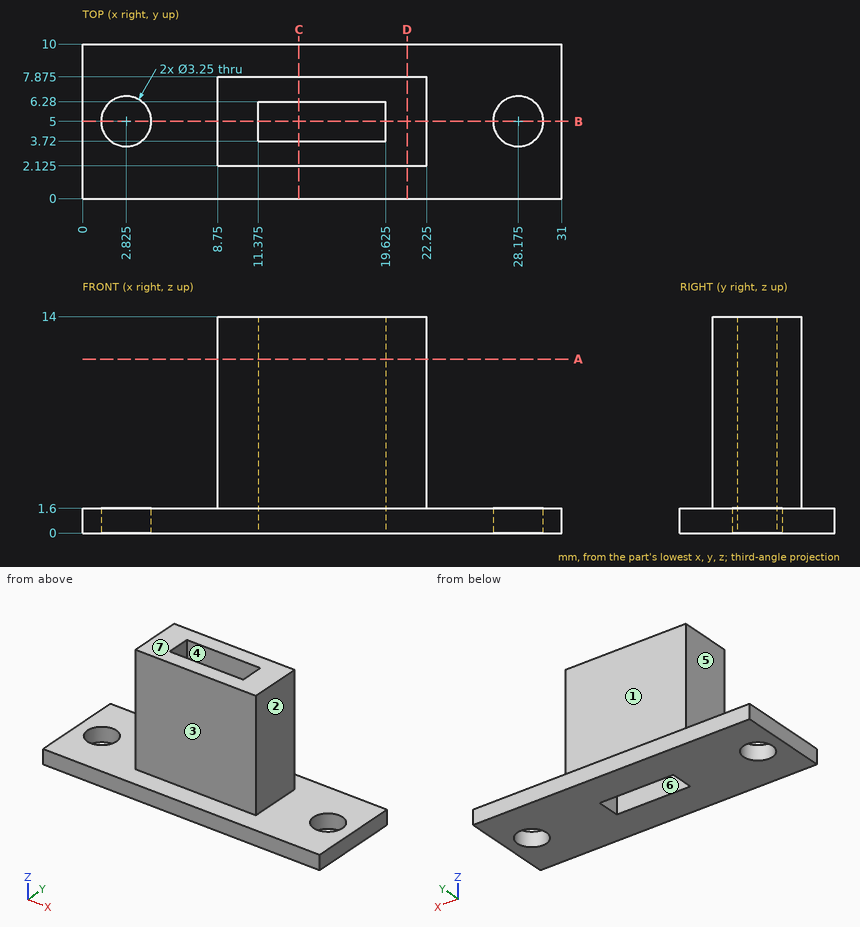
Can you work these out from the drawing? Everything is in mm from the part's minimum corner. A direction names the side the tool comes from. Round coordinates to 2 decimals unless told otherwise and drop trailing zeros. Write each loop counter-clockwise with the first axis right and the second up, starting at its lowest first coordinate (ties: lowest second). Pieces come first, ordered by that corner, then holes. Notation, with made-up numbers: M 5,16 L 59,16 A30 ccw 59,42 Z; hole C 35.5,1 d6. An arc over 180 degrees is marked long. Use a Markdown table: item, result.
Item 1: I want a section at D-D (x = 21). List the corners of the cut face in (y, z) for me (3 decimals), and give its area (3 significant figures).
Found:
| item | result |
|---|---|
| outline | M 0,0 L 10,0 L 10,1.6 L 7.875,1.6 L 7.875,14 L 2.125,14 L 2.125,1.6 L 0,1.6 Z |
| area | 87.3 mm2 |
Item 2: I want a section at C-C (x = 14). List the corners of the cut face in (y, z) for me (3 decimals), and give its area (3 significant figures).
Found:
| item | result |
|---|---|
| outline | M 0,0 L 3.72,0 L 3.72,14 L 2.125,14 L 2.125,1.6 L 0,1.6 Z; M 6.28,0 L 10,0 L 10,1.6 L 7.875,1.6 L 7.875,14 L 6.28,14 Z |
| area | 51.5 mm2 |
Item 3: Which directions (+Z, -Z, +X, -X, +Y, -Y) give clear straight access to the entire face, cutting with the end or side of a thin tool? Please do the marked faces 1, 2, 3 and 4.
Found:
| item | result |
|---|---|
| face 1 | +Z, +X, -X, +Y |
| face 2 | +Z, +X, +Y, -Y |
| face 3 | +Z, +X, -X, -Y |
| face 4 | +Z, -Z |
Item 4: For pin 1 Ø1.7 at (y, z) = (4.5, 6.5) entering from +X; pin 2 Ø6 at (x, z) = (13.5, 11) entering from -Y (3 decimals); pin 3 Ø2 at (y, z) = (5, 6.5) entering from -X, each with a flat end and sliding along its axis, tell me the tip position at first contact or that it passes through.
Found:
| item | result |
|---|---|
| pin 1 | stops at x = 22.25 |
| pin 2 | stops at y = 2.125 |
| pin 3 | stops at x = 8.75 |
Item 5: I want a section at B-B (y = 5). List the corners of the cut face in (x, z) for me (3 decimals).
Found:
| item | result |
|---|---|
| outline | M 0,0 L 1.2,0 L 1.2,1.6 L 0,1.6 Z; M 4.45,0 L 11.375,0 L 11.375,14 L 8.75,14 L 8.75,1.6 L 4.45,1.6 Z; M 19.625,0 L 26.55,0 L 26.55,1.6 L 22.25,1.6 L 22.25,14 L 19.625,14 Z; M 29.8,0 L 31,0 L 31,1.6 L 29.8,1.6 Z |
Item 6: We'd pull the mould along X, two halves only. Please class the marked faces 5, 6 and 7: released by +X, released by -X, zero draft, split by the parting line, or undercut.
Found:
| item | result |
|---|---|
| face 5 | released by -X |
| face 6 | undercut |
| face 7 | zero draft |
Item 7: I want a section at A-A (z = 11.25). List the corners of the cut face in (x, y) for me (3 decimals).
Found:
| item | result |
|---|---|
| outline | M 8.75,2.125 L 22.25,2.125 L 22.25,7.875 L 8.75,7.875 Z; hole M 11.375,3.72 L 19.625,3.72 L 19.625,6.28 L 11.375,6.28 Z |
Item 8: If I drill on line 1 along Y through (x, z) = (16, 2.75) (3 decimals); line 2 along X through (y, z) = (4.5, 8.75) (3 decimals); line 3 along Z through (x, y) = (28, 1.5), over which ranges is the centre line in solid material (lowest first)? Write a range as [from, to].
Found:
| item | result |
|---|---|
| line 1 | y = [2.125, 3.72], [6.28, 7.875] |
| line 2 | x = [8.75, 11.375], [19.625, 22.25] |
| line 3 | z = [0, 1.6] |
